For this review, take the finished solid that the model builds, in its own axes (mm). A direction names the side the tool comes from. Give positions to 0.01 mm unless a question says otherwise; leave off trailing zeros. Order: outer loops, then holes, each group sorted by start corner. A loop starts at its lowest first (then second) coordinate and runs counter-clockwise, first axis right, second up.
from build123d import *

# Parameters (mm, degrees)
SKETCH1_R           = 20
BOSS_EXTRUDE1_DEPTH = 10.16
SKETCH3_R           = 5
BOSS_EXTRUDE3_DEPTH = 30
CUT_EXTRUDE1_DEPTH  = 40.16
FILLET1_R           = 10
FILLET2_R           = 2


with BuildPart() as part:
    # Sketch1 → Boss-Extrude1 (new body)
    with BuildSketch(Plane(origin=(0, 0, 0), x_dir=(1, 0, 0), z_dir=(0, 1, 0))):
        Circle(SKETCH1_R)
    extrude(amount=BOSS_EXTRUDE1_DEPTH)

    # Sketch3 → Boss-Extrude3 (add)
    with BuildSketch(Plane.XZ):
        Circle(SKETCH3_R)
    extrude(amount=BOSS_EXTRUDE3_DEPTH)

    # Sketch5 → Cut-Extrude1 (cut)
    with BuildSketch(Plane.XZ.offset(30)):
        with BuildLine():
            Line((-1.983299019, 1.905), (1.983299019, 1.905))
            ThreePointArc((1.983299019, 1.905), (0, -2.75), (-1.983299019, 1.905))
        make_face()
    extrude(amount=-CUT_EXTRUDE1_DEPTH, mode=Mode.SUBTRACT)

    # Fillet1
    fillet1_edges = [part.edges().sort_by_distance(p)[0] for p in [
        (-5, 0, 0),
    ]]
    fillet(fillet1_edges, radius=FILLET1_R)

    # Fillet2
    fillet2_edges = [part.edges().sort_by_distance(p)[0] for p in [
        (-20, 0, 0),
        (-20, 10.16, 0),
    ]]
    fillet(fillet2_edges, radius=FILLET2_R)


solid = part.part
1) Tool access review of faces 1 (the face through (0, 10.16, 4)), 2 (the face through (-4, 0, -15)): name each direction out of +Z, -Z, +X, -X, +Y, -Y from which nothing blocks a thin tool from reaching the whole face with its end or side.
Answer sheet:
face 1: +Z, -Z, +X, -X, +Y
face 2: -Y
2) To check wall thickness, follow line 1 (Y direction, x = -3.5, z = 15); line 2 (X direction, y = -3, z = 0); line 3 (Z direction, x = -2.5, y = -11). State the ranges of each line that lie inside material, in increasing order.
Answer sheet:
line 1: y = 0 to 10.16
line 2: x = -7.86 to -2.75, 2.75 to 7.86
line 3: z = -4.33 to -1.15, 1.15 to 4.33
3) We need section D-D on y = -8.5. Give the boundary of the cut face in (x, z) (3 decimals).
Answer sheet:
outline: circle Ø10.226 at (0, 0); hole (-1.983, 1.905) arc R2.75 ccw (long way) to (1.983, 1.905) - close
4) We need section A-A on z = 0. Give the boundary of the cut face in (x, y), then the cut area to 3 significant figures.
Answer sheet:
outline: (-20, 2) arc R2 ccw to (-18, 0) - (-15, 0) arc R10 cw to (-5, -10) - (-5, -30) - (-2.75, -30) - (-2.75, 10.16) - (-18, 10.16) arc R2 ccw to (-20, 8.16) - close; (2.75, -30) - (5, -30) - (5, -10) arc R10 cw to (15, 0) - (18, 0) arc R2 ccw to (20, 2) - (20, 8.16) arc R2 ccw to (18, 10.16) - (2.75, 10.16) - close
area: 525 mm2
5) We need section B-B on x = 0. Give the boundary of the cut face in (y, z) (3 decimals).
Answer sheet:
outline: (-30, -5) - (-10, -5) arc R10 cw to (0, -15) - (0, -18) arc R2 ccw to (2, -20) - (8.16, -20) arc R2 ccw to (10.16, -18) - (10.16, -2.75) - (-30, -2.75) - close; (-30, 1.905) - (10.16, 1.905) - (10.16, 18) arc R2 ccw to (8.16, 20) - (2, 20) arc R2 ccw to (0, 18) - (0, 15) arc R10 cw to (-10, 5) - (-30, 5) - close
6) Draft analysis for pull direction Z (two halves, no side actions). For faces 3 (the face through (0.09, -10.2, -2.75)), 4 (the face through (-4.336, 5.037, 19.524)), 5 (the face through (-0.1, -30, 2.3)), 6 (the face through (0, -10, 1.905)), state which applies: +Z half, -Z half, draft (parallel to the pull), parting line (faces both ways), or undercut.
Answer sheet:
face 3: undercut
face 4: parting line
face 5: draft
face 6: undercut
7) We need section C-C on y = -15.5. Give the boundary of the cut face in (x, z) (3 decimals), then the cut area to 3 significant figures.
Answer sheet:
outline: circle Ø10 at (0, 0); hole (-1.983, 1.905) arc R2.75 ccw (long way) to (1.983, 1.905) - close
area: 57.1 mm2
8) Clearance check with flat-ended pins moving along their axes: pin 1 (2 mm diameter, centred on x = 1, y = -17.5, fed in from -Z); pin 2 (1 mm diameter, centred on y = -21, z = 0.5, fed in from +X); pin 3 (1 mm diameter, centred on x = -5, y = -22, fed in from +Z). State where each tip first meets the part, or that it passes through.
Answer sheet:
pin 1: stops at z = -5
pin 2: stops at x = 5
pin 3: stops at z = 2.18
